```python
from build123d import *

# Parameters (mm, degrees)
ESQUISSE1_W             = 178
ESQUISSE1_H             = 20
ESQUISSE1_W_2           = 20
BOSS_EXTRU_1_DEPTH      = 20
ESQUISSE3_W             = 17
ESQUISSE3_H             = 17
ENL_V_MAT_EXTRU_1_DEPTH = 178
ESQUISSE4_W             = 17
ESQUISSE4_H             = 17
ENL_V_MAT_EXTRU_2_DEPTH = 18.5
CHANFREIN1_SIZE         = 20
CHANFREIN1_SIZE2        = 11.547005384
ESQUISSE5_W             = 20
ESQUISSE5_H             = 0.5
ENL_V_MAT_EXTRU_3_DEPTH = 24
ESQUISSE6_R             = 1.6
ENL_V_MAT_EXTRU_4_DEPTH = 24
ESQUISSE7_R             = 3.2
ENL_V_MAT_EXTRU_5_DEPTH = 34


with BuildPart() as part:
    # Esquisse1 → Boss.-Extru.1 (new body)
    with BuildSketch(Plane.XY):
        Rectangle(ESQUISSE1_W, ESQUISSE1_H)
        with Locations((99, 0)):
            Rectangle(ESQUISSE1_W_2, ESQUISSE1_H)
    extrude(amount=BOSS_EXTRU_1_DEPTH)

    # Esquisse3 → Enlèv. mat.-Extru.1 (cut)
    with BuildSketch(Plane.ZY.offset(89)):
        with Locations((10, 0)):
            Rectangle(ESQUISSE3_W, ESQUISSE3_H)
    extrude(amount=-ENL_V_MAT_EXTRU_1_DEPTH, mode=Mode.SUBTRACT)

    # Esquisse4 → Enlèv. mat.-Extru.2 (cut)
    with BuildSketch(Plane.XY.offset(20)):
        with Locations((100.5, 0)):
            Rectangle(ESQUISSE4_W, ESQUISSE4_H)
    extrude(amount=-ENL_V_MAT_EXTRU_2_DEPTH, mode=Mode.SUBTRACT)

    # Chanfrein1
    chanfrein1_edges = [part.edges().sort_by_distance(p)[0] for p in [
        (109, 9.25, 20),
    ]]
    chanfrein1_side = [part.faces().sort_by_distance(p)[0] for p in [
        (2.875374557, 0, 20),
    ]]
    chamfer(chanfrein1_edges, length=CHANFREIN1_SIZE, length2=CHANFREIN1_SIZE2, reference=chanfrein1_side[0])

    # Esquisse5 → Enlèv. mat.-Extru.3 (cut)
    with BuildSketch(Plane(origin=(0, 0, 0), x_dir=(-1, 0, 0), z_dir=(0, 0, -1))):
        with Locations((-99, 9.75)):
            Rectangle(ESQUISSE5_W, ESQUISSE5_H)
        with Locations((-99, -9.75)):
            Rectangle(ESQUISSE5_W, ESQUISSE5_H)
    extrude(amount=-ENL_V_MAT_EXTRU_3_DEPTH, mode=Mode.SUBTRACT)

    # Esquisse6 → Enlèv. mat.-Extru.4 (cut)
    with BuildSketch(Plane(origin=(0, 0, 0), x_dir=(-1, 0, 0), z_dir=(0, 0, -1))):
        with Locations((-98.5, 6)):
            Circle(ESQUISSE6_R)
        with Locations((-98.5, -6)):
            Circle(ESQUISSE6_R)
    extrude(amount=-ENL_V_MAT_EXTRU_4_DEPTH, mode=Mode.SUBTRACT)

    # Esquisse7 → Enlèv. mat.-Extru.5 (cut)
    with BuildSketch(Plane.XZ.offset(10)):
        with Locations((-79, 10)):
            Circle(ESQUISSE7_R)
        with Locations((-41, 10)):
            Circle(ESQUISSE7_R)
    extrude(amount=-ENL_V_MAT_EXTRU_5_DEPTH, mode=Mode.SUBTRACT)


solid = part.part
```
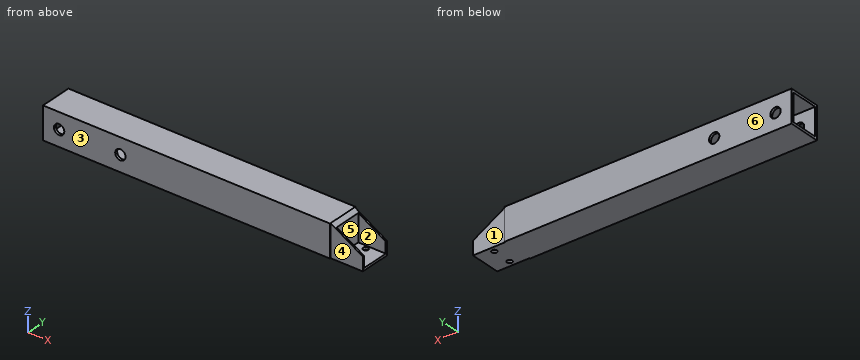
CAD build for the part. Positions are in the model's coordinates, mm. Face numbers are marked on the shaded views. A direction names the side the tool comes from. Round coordinates to 2 decimals unless told otherwise and drop trailing zeros. Loops run counter-clockwise (first coordinate to the right, second up) from the corner with the lowest first, then second, coordinate; pieces in that order, holes last. Notation, with made-up numbers: M 52,83 L 82,83 A32 cw 82,117 Z; hole C -9.75,21 d4. An arc over 180 degrees is marked long. Use a Markdown table: item, result. Add a question column.
(1) Drill centre lines: line 1 (Y direction, x = 98.5, z = 0.4); line 2 (Z direction, x = 63, y = -2.5); line 3 (Y direction, x = 15, z = 16.5). Where is each one in solid material? Low to high.
(2) Cut at A-A (x = -41). Give the cut face in (y, z).
(3) Which spindle directions (+Z, -Z, +X, -X, +Y, -Y) get a long thin tool onto all of the face, cutting with end or side? Do the marked faces 1, 2 and 3. Say none if no direction does.
(4) Pull direction Y, two halves, no side cores. Call the marked faces 4, 5 and 6: +Y half, -Y half, draft (parallel to the pull), parting line (faces both ways), or undercut.
(5) Cut at C-C (y = 2.75). Give the cut face in (x, z), and give its area (3 significant figures).
(6) Cut at B-B (x = -9). Give the cut face in (y, z), and give its area (3 significant figures).
(7) Flat gauge pins, fed straight in: pin 1 (8.5 mm diameter, centred on x = -41, z = 10, fed in from -Y); pin 2 (4 mm diameter, centred on y = -5, z = 6.5, fed in from +X); pin 3 (6 mm diameter, centred on x = 97.5, z = 14.5, fed in from -Y). Where does each tip first touch, or does it go through?
Geometry says:
| question | item | result |
|---|---|---|
| 1 | line 1 | y = -9.5 to -7.6, -4.4 to 4.4, 7.6 to 9.5 |
| 1 | line 2 | z = 0 to 1.5, 18.5 to 20 |
| 1 | line 3 | y = -10 to -8.5, 8.5 to 10 |
| 2 | outline | M -10,0 L 10,0 L 10,6.8 L 8.5,6.8 L 8.5,1.5 L -8.5,1.5 L -8.5,6.8 L -10,6.8 Z; M -10,13.2 L -8.5,13.2 L -8.5,18.5 L 8.5,18.5 L 8.5,13.2 L 10,13.2 L 10,20 L -10,20 Z |
| 3 | face 1 | +Z, -Z, +X, +Y |
| 3 | face 2 | +Z, +X |
| 3 | face 3 | +Z, -Z, +X, -X, -Y |
| 4 | face 4 | -Y half |
| 4 | face 5 | undercut |
| 4 | face 6 | +Y half |
| 5 | outline | M -89,0 L 109,0 L 109,1.5 L 92,1.5 L 92,18.27 L 89,20 L -89,20 L -89,18.5 L 89,18.5 L 89,1.5 L -89,1.5 Z |
| 5 | area | 617 mm² |
| 6 | outline | M -10,0 L 10,0 L 10,20 L -10,20 Z; hole M -8.5,1.5 L 8.5,1.5 L 8.5,18.5 L -8.5,18.5 Z |
| 6 | area | 111 mm² |
| 7 | pin 1 | stops at y = -10 |
| 7 | pin 2 | stops at x = 92 |
| 7 | pin 3 | stops at y = -9.5 |
